Drawing for the job (mm, zero at the part's lowest x, y, z). A direction names the side the tool comes from. Round coordinates to 2 decimals unless told otherwise and drop trailing zeros. Write each loop counter-clockwise with the first axis right and the second up, starting at its lowest first coordinate (ties: lowest second). Pieces come first, ordered by that corner, then holes. Notation, with made-up numbers: M -25,65.25 L -13,65.25 A20 cw -13,97.25 Z; hole C 31.5,66.5 d4. An arc over 180 degrees is marked long. Use a Markdown table: item, result.
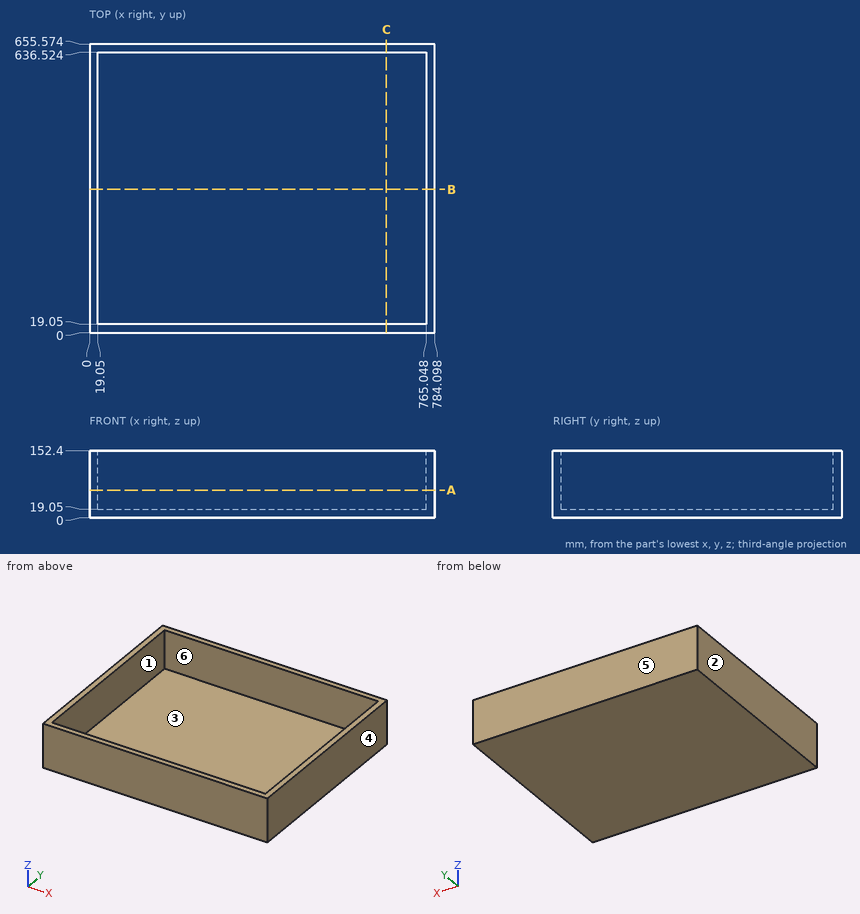
Q1. Two-plate mould, pull along Y, no slides. Class the marked faces 3, 4, 5 and 6: +Y half, -Y half, draft (parallel to the pull), parting line (faces both ways), or undercut.
Response values:
| item | result |
|---|---|
| face 3 | undercut |
| face 4 | draft |
| face 5 | +Y half |
| face 6 | undercut |
Q2. Drop a flat-ended pin along its axis: P1, Ø4, axis at x = 607.5, y = 167, coming from the +Z side. Give the stop position or say it passes through.
Response values:
| item | result |
|---|---|
| P1 | stops at z = 19.05 |
Q3. Cut at C-C on x = 674. Give the cut face in (y, z), and give its area (3 significant figures).
Response values:
| item | result |
|---|---|
| outline | M 0,0 L 655.57,0 L 655.57,152.4 L 636.52,152.4 L 636.52,19.05 L 19.05,19.05 L 19.05,152.4 L 0,152.4 Z |
| area | 17,600 mm2 |
Q4. Drill centre lines: L1, parallel to X at y = 101, z = 34.5; L2, parallel to Y at x = 569.5, z = 61; L3, parallel to Z at x = 484, y = 574.5. Where is each one in solid material? Low to high.
Response values:
| item | result |
|---|---|
| L1 | x = 0 to 19.05, 765.05 to 784.1 |
| L2 | y = 0 to 19.05, 636.52 to 655.57 |
| L3 | z = 0 to 19.05 |
Q5. Cut at B-B on y = 325.5. Give the cut face in (x, z).
Response values:
| item | result |
|---|---|
| outline | M 0,0 L 784.1,0 L 784.1,152.4 L 765.05,152.4 L 765.05,19.05 L 19.05,19.05 L 19.05,152.4 L 0,152.4 Z |
Q6. Which spindle directions (+Z, -Z, +X, -X, +Y, -Y) get a long thin tool onto all of the face, cutting with end or side? Do the marked faces 1 and 2. Say none if no direction does.
Response values:
| item | result |
|---|---|
| face 1 | +Z |
| face 2 | +Z, -Z, -X, +Y, -Y |
Q7. Cut at A-A on z = 63. Give the cut face in (x, y).
Response values:
| item | result |
|---|---|
| outline | M 0,0 L 784.1,0 L 784.1,655.57 L 0,655.57 Z; hole M 19.05,19.05 L 765.05,19.05 L 765.05,636.52 L 19.05,636.52 Z |
